Check sheet for the modelled part. Datum: model origin and axes. Units: mm. Coordinates: 2 decimals unless noted, no trailing zeros. Loops run counter-clockwise (first coordinate to the right, second up) from the corner with the lowest first, then second, coordinate; pieces in that order, holes last. Notation, with made-up numbers: (81.25, -31) - (107.25, -31) arc R18 cw to (107.25, 2) - close; hole circle Ø2 at (27.5, 27). An arc over 180 degrees is marked (long way). Answer as a JSON object with one key per item and string values. Group by question number.
from build123d import *

# Parameters (mm, degrees)
SKETCH1_R           = 15
SKETCH1_R_2         = 13.5
BOSS_EXTRUDE1_DEPTH = 5.5
SKETCH2_R           = 0.5
CUT_EXTRUDE1_DEPTH  = 5.5
CIRPATTERN1_COUNT   = 6
SCALE1_SCALE        = 5


with BuildPart() as part:
    # Sketch1 → Boss-Extrude1 (new body)
    with BuildSketch(Plane(origin=(0, 0, 0), x_dir=(1, 0, 0), z_dir=(0, 1, 0))):
        with Locations(Location((0, 0, 0), (0, 0, 270))):
            Circle(SKETCH1_R)
        with Locations(Location((0, 0, 0), (0, 0, 270))):
            Circle(SKETCH1_R_2, mode=Mode.SUBTRACT)
    extrude(amount=BOSS_EXTRUDE1_DEPTH)

    # Sketch2 → Cut-Extrude1 (cut)
    with BuildSketch(Plane(origin=(0, 5.5, 0), x_dir=(1, 0, 0), z_dir=(0, 1, 0))):
        with Locations(Location((0, 14.2, 0), (0, 0, 270))):
            Circle(SKETCH2_R)
    cut_extrude1 = extrude(amount=-CUT_EXTRUDE1_DEPTH, mode=Mode.SUBTRACT)

    # CirPattern1: Cut-Extrude1 ×6 about axis
    cirpattern1_axis = Axis((0, 0, 0), (0, 1, 0))
    for i in range(1, CIRPATTERN1_COUNT):
        add(cut_extrude1.rotate(cirpattern1_axis, i * 360 / CIRPATTERN1_COUNT), mode=Mode.SUBTRACT)


with BuildPart() as part_1:
    # Scale1: scaled about (0, 2.75, 0)
    add(part.part.scale(SCALE1_SCALE).moved(Location((0, -11, 0))))


solid = part_1.part
1. Sectioned sample at B-B on z = -71. Record the cut outline in (x, y), plus the area to 3 significant figures.
2. Sectioned sample at A-A on x = 0. Record the cut outline in (y, z).
3. Material ranges on line 1 (X direction, y = -3, z = 0); line 2 (X direction, y = 8.75, z = -35.5); line 3 (Z direction, x = -57, y = 10.25), recorded low to high.
4. Sectioned sample at D-D on z = 0. Record the cut outline in (x, y), plus the area to 4 significant figures.
5. Sectioned sample at C-C on y = -2. Record the cut outline in (x, z), plus the area to 3 significant figures.
6. Release check for a two-part mould opening along X. For faces 1 (the face through (-59.884, 2.557, 31.147)), 2 (the face through (1.5, 2.9, 73)), 3 (the face through (-55.2, -11, -39.2)), 4 (the face through (-45.636, 2.557, -59.517)) record: released by +X, released by -X, zero draft, split by the parting line, or undercut.
7. Gauge pin test, flat ends, axial feed: pin 1 (2 mm diameter, centred on x = 4.5, y = -6.5, fed in from -Z); pin 2 (1.5 mm diameter, centred on y = -2.5, z = -51.5, fed in from -X); pin 3 (1 mm diameter, centred on x = 53.5, y = -5, fed in from -Z). Record the tip position at first contact, or that the pin passes through.
Answers follow:
{
 "1": {"outline": "(-24.17, -11) - (-2.5, -11) - (-2.5, 16.5) - (-24.17, 16.5) - close; (2.5, -11) - (24.17, -11) - (24.17, 16.5) - (2.5, 16.5) - close", "area": "1,190 mm^2"},
 "2": {"outline": "(-11, -75) - (16.5, -75) - (16.5, -73.5) - (-11, -73.5) - close; (-11, -68.5) - (16.5, -68.5) - (16.5, -67.5) - (-11, -67.5) - close; (-11, 67.5) - (16.5, 67.5) - (16.5, 68.5) - (-11, 68.5) - close; (-11, 73.5) - (16.5, 73.5) - (16.5, 75) - (-11, 75) - close"},
 "3": {"line 1": "x = -75 to -67.5, 67.5 to 75", "line 2": "x = -66.07 to -63.99, -58.99 to -57.41, 57.41 to 58.99, 63.99 to 66.07", "line 3": "z = -48.74 to -36.16, 36.16 to 48.74"},
 "4": {"outline": "(-75, -11) - (-67.5, -11) - (-67.5, 16.5) - (-75, 16.5) - close; (67.5, -11) - (75, -11) - (75, 16.5) - (67.5, 16.5) - close", "area": "412.5 mm^2"},
 "5": {"outline": "circle Ø150 at (0, 0); hole circle Ø135 at (0, 0); hole circle Ø5 at (-61.49, -35.5); hole circle Ø5 at (-61.49, 35.5); hole circle Ø5 at (0, -71); hole circle Ø5 at (0, 71); hole circle Ø5 at (61.49, -35.5); hole circle Ø5 at (61.49, 35.5)", "area": "3,240 mm^2"},
 "6": {"face 1": "undercut", "face 2": "undercut", "face 3": "zero draft", "face 4": "split by the parting line"},
 "7": {"pin 1": "stops at z = -74.92", "pin 2": "stops at x = -55.22", "pin 3": "stops at z = -53.07"}
}
